from build123d import *

# Parameters (mm, degrees)
SKETCH1_W                          = 120.65
SKETCH1_H                          = 25.4
BOSS_EXTRUDE1_DEPTH                = 3.175
CUT_EXTRUDE1_REACH                 = 107.281
SKETCH4_R                          = 3.5
F_8_CLEARANCE_HOLE1_D              = 4.4958
FILLET3_R                          = 3.175
CUT_EXTRUDE3_REACH                 = 98.693
SKETCH12_W                         = 6.35
SKETCH12_H                         = 15.24
TAP_DRILL_FOR_8_32_TAP1_D          = 3.4544
TAP_DRILL_FOR_8_32_TAP1_DEPTH      = 12.7
TAP_DRILL_FOR_8_32_TAP1_TIP        = 1.037806461
TAP_DRILL_FOR_8_32_TAP2_AT_2_COUNT = 2
TAP_DRILL_FOR_8_32_TAP2_AT_2_PITCH = 47.625
TAP_DRILL_FOR_8_32_TAP2_AT_3_COUNT = 2
TAP_DRILL_FOR_8_32_TAP2_AT_3_PITCH = 66.675
TAP_DRILL_FOR_8_32_TAP2_AT_4_COUNT = 2
TAP_DRILL_FOR_8_32_TAP2_AT_4_PITCH = 114.3


# Read off the part's stored shape, not the designer's step: AdvancedHole1
with BuildPart() as part:
    # Sketch1 → Boss-Extrude1 (new, symmetric)
    with BuildSketch(Plane(origin=(0, 0, 0), x_dir=(0, 0, -1), z_dir=(1, 0, 0))):
        Rectangle(SKETCH1_W, SKETCH1_H)
        Polygon((-60.325, 12.7), (-104.319090512, -12.7), (-60.325, -12.7), align=None)
    extrude(amount=BOSS_EXTRUDE1_DEPTH, both=True)

    # Sketch4 → Cut-Extrude1 (cut, up to next)
    with BuildSketch(Plane(origin=(3.175, 0, 0), x_dir=(0, 0, -1), z_dir=(1, 0, 0)), mode=Mode.PRIVATE) as cut_extrude1_sk1:
        with Locations((-39.37, 0)):
            Circle(SKETCH4_R)
    cut_extrude1_tool1 = extrude(cut_extrude1_sk1.sketch, amount=-CUT_EXTRUDE1_REACH, mode=Mode.PRIVATE) & part.part
    # Sketch4 → Cut-Extrude1 (cut, up to next)
    with BuildSketch(Plane(origin=(3.175, 0, 0), x_dir=(0, 0, -1), z_dir=(1, 0, 0)), mode=Mode.PRIVATE) as cut_extrude1_sk2:
        with Locations((39.37, 0)):
            Circle(SKETCH4_R)
    cut_extrude1_tool2 = extrude(cut_extrude1_sk2.sketch, amount=-CUT_EXTRUDE1_REACH, mode=Mode.PRIVATE) & part.part
    add(cut_extrude1_tool1.solids().sort_by_distance((3.175, 0, 39.37))[0], mode=Mode.SUBTRACT)
    add(cut_extrude1_tool2.solids().sort_by_distance((3.175, 0, -39.37))[0], mode=Mode.SUBTRACT)

    # AdvancedHole1 outline → AdvancedHole1 (revolve, cut)
    with BuildSketch(Plane(origin=(0, -8.5, -39.37), x_dir=(0, 1, 0), z_dir=(0, 0, -1))):
        Polygon((0.889, 2.6528283), (1.5113, 3.175), (0, 3.175), (0, -3.175), (1.7, -3.175), (1.7, 2.6528283), align=None)
    revolve(axis=Axis((0, -8.5, -39.37), (1, 0, 0)), mode=Mode.SUBTRACT)

    # AdvancedHole1 2 outline → AdvancedHole1 2 (revolve, cut)
    with BuildSketch(Plane(origin=(0, 8.5, -39.37), x_dir=(0, 1, 0), z_dir=(0, 0, -1))):
        Polygon((0.889, 2.6528283), (1.5113, 3.175), (0, 3.175), (0, -3.175), (1.7, -3.175), (1.7, 2.6528283), align=None)
    revolve(axis=Axis((0, 8.5, -39.37), (1, 0, 0)), mode=Mode.SUBTRACT)

    # AdvancedHole1 3 outline → AdvancedHole1 3 (revolve, cut)
    with BuildSketch(Plane(origin=(0, -8.5, 39.37), x_dir=(0, 1, 0), z_dir=(0, 0, -1))):
        Polygon((0.889, 2.6528283), (1.5113, 3.175), (0, 3.175), (0, -3.175), (1.7, -3.175), (1.7, 2.6528283), align=None)
    revolve(axis=Axis((0, -8.5, 39.37), (1, 0, 0)), mode=Mode.SUBTRACT)

    # AdvancedHole1 4 outline → AdvancedHole1 4 (revolve, cut)
    with BuildSketch(Plane(origin=(0, 8.5, 39.37), x_dir=(0, 1, 0), z_dir=(0, 0, -1))):
        Polygon((0.889, 2.6528283), (1.5113, 3.175), (0, 3.175), (0, -3.175), (1.7, -3.175), (1.7, 2.6528283), align=None)
    revolve(axis=Axis((0, 8.5, 39.37), (1, 0, 0)), mode=Mode.SUBTRACT)

    # #8 Clearance Hole1 (through all)
    with Locations(Plane(origin=(3.175, 0, 0), x_dir=(0, 0, -1), z_dir=(1, 0, 0))):
        with Locations((-15.875, 7.9375), (-15.875, -7.9375), (15.875, -7.9375), (15.875, 7.9375)):
            Hole(F_8_CLEARANCE_HOLE1_D / 2)

    # Fillet3
    fillet3_edges = [part.edges().sort_by_distance(p)[0] for p in [
        (0, -12.7, 104.319090512),
    ]]
    fillet(fillet3_edges, radius=FILLET3_R)

    # Sketch12 → Cut-Extrude3 (cut, up to next)
    with BuildSketch(Plane(origin=(3.175, 0, 0), x_dir=(0, 0, -1), z_dir=(1, 0, 0)), mode=Mode.PRIVATE) as cut_extrude3_sk1:
        with Locations((-57.15, 0)):
            Rectangle(SKETCH12_W, SKETCH12_H)
    cut_extrude3_tool1 = extrude(cut_extrude3_sk1.sketch, amount=-CUT_EXTRUDE3_REACH, mode=Mode.PRIVATE) & part.part
    # Sketch12 → Cut-Extrude3 (cut, up to next)
    with BuildSketch(Plane(origin=(3.175, 0, 0), x_dir=(0, 0, -1), z_dir=(1, 0, 0)), mode=Mode.PRIVATE) as cut_extrude3_sk2:
        with Locations((57.15, 0)):
            Rectangle(SKETCH12_W, SKETCH12_H)
    cut_extrude3_tool2 = extrude(cut_extrude3_sk2.sketch, amount=-CUT_EXTRUDE3_REACH, mode=Mode.PRIVATE) & part.part
    add(cut_extrude3_tool1.solids().sort_by_distance((3.175, 0, 57.15))[0], mode=Mode.SUBTRACT)
    add(cut_extrude3_tool2.solids().sort_by_distance((3.175, 0, -57.15))[0], mode=Mode.SUBTRACT)

    # Tap Drill for #8-32 Tap1
    with Locations(Plane(origin=(0, 35.646491242, 20.580511314), x_dir=(1, 0, 0), z_dir=(0, 0.8660254037844417, 0.4999999999999949))):
        with Locations((0, -64.942982483), (0, -55.417982483)):
            Hole(TAP_DRILL_FOR_8_32_TAP1_D / 2, depth=TAP_DRILL_FOR_8_32_TAP1_DEPTH)
            with Locations((0, 0, -(TAP_DRILL_FOR_8_32_TAP1_DEPTH + TAP_DRILL_FOR_8_32_TAP1_TIP / 2))):  # 118° drill point
                Cone(0, TAP_DRILL_FOR_8_32_TAP1_D / 2, TAP_DRILL_FOR_8_32_TAP1_TIP, mode=Mode.SUBTRACT)

    # Sketch20 → Tap Drill for #8-32 Tap2 (revolve, cut)
    with BuildSketch(Plane(origin=(0, 12.7, 57.15), x_dir=(0, 0, 1), z_dir=(1, 0, 0))):
        Polygon((0, 0), (0, 13.737806461), (1.7272, 12.7), (1.7272, 0), align=None)
    tap_drill_for_8_32_tap2 = revolve(axis=Axis((0, 19.05, 57.15), (0, -1, 0)), mode=Mode.SUBTRACT)

    # Tap Drill for #8-32 Tap2 at 2: Tap Drill for #8-32 Tap2 ×2
    with Locations(*[(0, 0, -i * TAP_DRILL_FOR_8_32_TAP2_AT_2_PITCH) for i in range(1, TAP_DRILL_FOR_8_32_TAP2_AT_2_COUNT)]):
        add(tap_drill_for_8_32_tap2, mode=Mode.SUBTRACT)

    # Tap Drill for #8-32 Tap2 at 3: Tap Drill for #8-32 Tap2 ×2
    with Locations(*[(0, 0, -i * TAP_DRILL_FOR_8_32_TAP2_AT_3_PITCH) for i in range(1, TAP_DRILL_FOR_8_32_TAP2_AT_3_COUNT)]):
        add(tap_drill_for_8_32_tap2, mode=Mode.SUBTRACT)

    # Tap Drill for #8-32 Tap2 at 4: Tap Drill for #8-32 Tap2 ×2
    with Locations(*[(0, 0, -i * TAP_DRILL_FOR_8_32_TAP2_AT_4_PITCH) for i in range(1, TAP_DRILL_FOR_8_32_TAP2_AT_4_COUNT)]):
        add(tap_drill_for_8_32_tap2, mode=Mode.SUBTRACT)

    # Mirror1: Tap Drill for #8-32 Tap2 across plane
    add(tap_drill_for_8_32_tap2.mirror(Plane.ZX), mode=Mode.SUBTRACT)

    # Mirror1 copy 1 sketch → Mirror1 copy 1 (revolve, cut)
    with BuildSketch(Plane(origin=(0, -12.7, 9.525), x_dir=(0, 0, 1), z_dir=(1, 0, 0))):
        Polygon((0, 0), (0, -13.737806461), (1.7272, -12.7), (1.7272, 0), align=None)
    revolve(axis=Axis((0, -19.05, 9.525), (0, -1, 0)), mode=Mode.SUBTRACT)

    # Mirror1 copy 2 sketch → Mirror1 copy 2 (revolve, cut)
    with BuildSketch(Plane(origin=(0, -12.7, -9.525), x_dir=(0, 0, 1), z_dir=(1, 0, 0))):
        Polygon((0, 0), (0, -13.737806461), (1.7272, -12.7), (1.7272, 0), align=None)
    revolve(axis=Axis((0, -19.05, -9.525), (0, -1, 0)), mode=Mode.SUBTRACT)

    # Mirror1 copy 3 sketch → Mirror1 copy 3 (revolve, cut)
    with BuildSketch(Plane(origin=(0, -12.7, -57.15), x_dir=(0, 0, 1), z_dir=(1, 0, 0))):
        Polygon((0, 0), (0, -13.737806461), (1.7272, -12.7), (1.7272, 0), align=None)
    revolve(axis=Axis((0, -19.05, -57.15), (0, -1, 0)), mode=Mode.SUBTRACT)


solid = part.part
For this review, take the finished solid that the model builds, in its own axes (mm). A direction names the side the tool comes from. Round coordinates to 2 decimals unless told otherwise and drop trailing zeros. Order: outer loops, then holes, each group sorted by start corner. A loop starts at its lowest first (then second) coordinate and runs counter-clockwise, first axis right, second up. Notation, with made-up numbers: M 71.5,60 L 121.5,60 A31 ccw 121.5,99 Z; hole C 29,18 d9. An arc over 180 degrees is marked long. Write each question's results on one line, items separated by ' | '. Start each with the question number.
1. Add section D-D (z = 82). State the section outline as (x, y) points (3 decimals), then the cut area to 3 significant figures.
2. Clearance check with flat-ended pins moving along their axes: pin 1 Ø3 at (x, z) = (0, 9.525) entering from +Y; pin 2 Ø1 at (y, z) = (8.5, -38.5) entering from -X; pin 3 Ø3 at (x, y) = (-1, -2.5) entering from -Z (3 decimals); pin 4 Ø1 at (x, y) = (-0.5, 7.5) entering from +Z. State where each tip first meets the part, or that it passes through.
3. Draft analysis for pull direction X (two halves, no side actions). For faces 1 (the face through (-0.04, -8.42, 69.79)), 2 (the face through (2.653, 8.5, -40.5)), 3 (the face through (0.04, 1.05, -42.71)), state which applies: pulls with the +X half, pulls with the -X half, needs draft (parallel to the pull), parting line crosses it, or undercut.
4. Tool access review of faces 4 (the face through (-1.4, 7.62, 55.8)), 5 (the face through (2.653, -9, 38)), 6 (the face through (-0.519, 10.196, -55.503)), 7 (the face through (-1, -7.62, -59)): name each direction out of +Z, -Z, +X, -X, +Y, -Y from which nothing blocks a thin tool from reaching the whole face with its end or side.
5. To check wall thickness, follow L1, parallel to Y at x = -1.5, z = 56; L2, parallel to Z at x = 2, y = 8.25 (3 decimals); L3, parallel to Y at x = 0.75, z = 39. State the ranges of each line that lie inside material, in increasing order. Write a range as [from, to].
6. Add section B-B (z = 16.5). State the section outline as (x, y) points (3 decimals), then the cut area to 3 significant figures.
7. Add section A-A (z = 57.15). State the section outline as (x, y) points (3 decimals).
8. Add section C-C (z = -39.37). State the section outline as (x, y) points (3 decimals).
Output values:
1) outline: M -3.175,-12.7 L 3.175,-12.7 L 3.175,0.186 L -3.175,0.186 Z | area: 81.8 mm^2
2) pin 1: through | pin 2: x = 2.65 | pin 3: z = -53.975 | pin 4: z = 70.2
3) face 1: undercut | face 2: pulls with the -X half | face 3: needs draft
4) face 4: +X, -X | face 5: -X | face 6: +Y, -Y | face 7: -Z, +X, -X
5) L1: [-12.7, -7.62], [7.62, 12.7] | L2: [-60.325, -41.052], [-37.688, -18.101], [-13.649, 13.649], [18.101, 37.688], [41.052, 68.033] | L3: [-12.7, -10.16], [-6.84, -3.48], [3.48, 6.84], [10.16, 12.7]
6) outline: M -3.175,-12.7 L 3.175,-12.7 L 3.175,-10.097 L -3.175,-10.097 Z; M -3.175,-5.778 L 3.175,-5.778 L 3.175,5.778 L -3.175,5.778 Z; M -3.175,10.097 L 3.175,10.097 L 3.175,12.7 L -3.175,12.7 Z | area: 106 mm^2
7) outline: M -3.175,-12.7 L -1.727,-12.7 L -1.727,-7.62 L -3.175,-7.62 Z; M -3.175,7.62 L -1.727,7.62 L -1.727,12.7 L -3.175,12.7 Z; M 1.727,-12.7 L 3.175,-12.7 L 3.175,-7.62 L 1.727,-7.62 Z; M 1.727,7.62 L 3.175,7.62 L 3.175,12.7 L 1.727,12.7 Z
8) outline: M -3.175,-12.7 L 3.175,-12.7 L 3.175,-10.011 L 2.653,-9.389 L 2.653,-10.2 L -3.175,-10.2 Z; M -3.175,-6.8 L 2.653,-6.8 L 2.653,-7.611 L 3.175,-6.989 L 3.175,-3.5 L -3.175,-3.5 Z; M -3.175,3.5 L 3.175,3.5 L 3.175,6.989 L 2.653,7.611 L 2.653,6.8 L -3.175,6.8 Z; M -3.175,10.2 L 2.653,10.2 L 2.653,9.389 L 3.175,10.011 L 3.175,12.7 L -3.175,12.7 Z
